Geometry: final body of the model. Coordinates: model frame, mm. A direction names the side the tool comes from. Round coordinates to 2 decimals unless told otherwise and drop trailing zeros. Loops run counter-clockwise (first coordinate to the right, second up) from the corner with the lowest first, then second, coordinate; pieces in that order, holes last. Notation, with made-up numbers: (-33, 74) - (-14, 74) arc R20 cw to (-14, 90) - close; hole circle Ø4 at (68, 14.5). An arc over 180 degrees is marked (long way). Use CSV: the item, a comma, the result in double quotes.
from build123d import *

# Parameters (mm, degrees)
F0_W     = 120
F0_H     = 67.5
F1_DEPTH = 1
F2_R     = 2.55
F3_DEPTH = 25
F4_R     = 3
F5_R     = 2.55
F6_DEPTH = 25


with BuildPart() as f1:
    # F0 (on Top) → F1 (new body)
    with BuildSketch(Plane.XY):
        with Locations((60, -33.75)):
            Rectangle(F0_W, F0_H)
    extrude(amount=F1_DEPTH)

    # F2 (on face) → F3 (cut)
    with BuildSketch(Plane.XY.offset(1)):
        with BuildLine():
            Line((105.25, -23.75), (14.75, -23.75))
            ThreePointArc((14.75, -23.75), (12.62868, -24.62868), (11.75, -26.75))
            Line((11.75, -26.75), (11.75, -40.75))
            ThreePointArc((11.75, -40.75), (12.62868, -42.87132), (14.75, -43.75))
            Line((14.75, -43.75), (105.25, -43.75))
            ThreePointArc((105.25, -43.75), (107.37132, -42.87132), (108.25, -40.75))
            Line((108.25, -40.75), (108.25, -26.75))
            ThreePointArc((108.25, -26.75), (107.37132, -24.62868), (105.25, -23.75))
        make_face()
        with Locations((7.5, -4.5)):
            Circle(F2_R)
        with Locations((7.5, -63)):
            Circle(F2_R)
        with Locations((25, -4.5)):
            Circle(F2_R)
        with Locations((25, -63)):
            Circle(F2_R)
        with Locations((42.5, -4.5)):
            Circle(F2_R)
        with Locations((42.5, -63)):
            Circle(F2_R)
        with Locations((60, -4.5)):
            Circle(F2_R)
        with Locations((60, -63)):
            Circle(F2_R)
        with Locations((77.5, -4.5)):
            Circle(F2_R)
        with Locations((77.5, -63)):
            Circle(F2_R)
        with Locations((95, -4.5)):
            Circle(F2_R)
        with Locations((95, -63)):
            Circle(F2_R)
        with Locations((112.5, -4.5)):
            Circle(F2_R)
        with Locations((112.5, -63)):
            Circle(F2_R)
    extrude(amount=-F3_DEPTH, mode=Mode.SUBTRACT)

    # F4
    f4_edges = [f1.edges().sort_by_distance(p)[0] for p in [
        (0, 0, 0.5),
        (0, -67.5, 0.5),
        (120, 0, 0.5),
        (120, -67.5, 0.5),
    ]]
    fillet(f4_edges, radius=F4_R)

    # F5 (on face) → F6 (cut)
    with BuildSketch(Plane.XY.offset(1)):
        with Locations((115, -45.25)):
            Circle(F5_R)
        with Locations((115, -22.25)):
            Circle(F5_R)
        with Locations((5, -45.25)):
            Circle(F5_R)
        with Locations((5, -22.25)):
            Circle(F5_R)
    extrude(amount=-F6_DEPTH, mode=Mode.SUBTRACT)


solid = f1.part
Item 1: Pin query (flat end, axial travel): P1, Ø4.5, axis at x = 112.5, y = -4.5, coming from the +Z side. Return the tip coordinate at first contact, or that it passes through.
Final values:
P1,"passes through"
Item 2: Section C-C on x = 31.5. Return the cut outline in (y, z).
Final values:
outline,"(-67.5, 0) - (-43.75, 0) - (-43.75, 1) - (-67.5, 1) - close; (-23.75, 0) - (0, 0) - (0, 1) - (-23.75, 1) - close"
Item 3: Reachability of faces 1 (the cylindrical face through (107.35, -42.89, 0.51)), 2 (the flat face through (59, -18, 1)) from +Z, -Z, +X, -X, +Y, -Y: full face, straight path, thin tool, end or side. Return the list, or none.
Final values:
face 1,"+Z, -Z"
face 2,"+Z, +X, -X, +Y, -Y"
Item 4: Mould query, pull axis Y, two halves, no side actions, for faces 3 (the cylindrical face through (0.86, -66.6, 0.51)), 4 (the cylindrical face through (0.86, -0.9, 0.51)), 5 (the cylindrical face through (78.87, -60.85, 0.51)). Classes: released by +Y, released by -Y, zero draft, split by the parting line, or undercut.
Final values:
face 3,"released by -Y"
face 4,"released by +Y"
face 5,"undercut"
Item 5: Section D-D on y = -22.25. Return the cut outline in (x, z), plus the area to 3 significant figures.
Final values:
outline,"(0, 0) - (2.45, 0) - (2.45, 1) - (0, 1) - close; (7.55, 0) - (112.45, 0) - (112.45, 1) - (7.55, 1) - close; (117.55, 0) - (120, 0) - (120, 1) - (117.55, 1) - close"
area,"110 mm²"
Item 6: Section A-A on x = 95. Return the cut outline in (y, z).
Final values:
outline,"(-67.5, 0) - (-65.55, 0) - (-65.55, 1) - (-67.5, 1) - close; (-60.45, 0) - (-43.75, 0) - (-43.75, 1) - (-60.45, 1) - close; (-23.75, 0) - (-7.05, 0) - (-7.05, 1) - (-23.75, 1) - close; (-1.95, 0) - (0, 0) - (0, 1) - (-1.95, 1) - close"
Item 7: Material intervals for line 1 (Y direction, x = 60, z = 0.2); line 2 (Y direction, x = 33.5, z = 0.3); line 3 (X direction, y = -27.5, z = 0.15), sorted ascending.
Final values:
line 1,"y = -67.5 to -65.55, -60.45 to -43.75, -23.75 to -7.05, -1.95 to 0"
line 2,"y = -67.5 to -43.75, -23.75 to 0"
line 3,"x = 0 to 11.75, 108.25 to 120"
Item 8: Section B-B on y = -32.5. Return the cut outline in (x, z).
Final values:
outline,"(0, 0) - (11.75, 0) - (11.75, 1) - (0, 1) - close; (108.25, 0) - (120, 0) - (120, 1) - (108.25, 1) - close"
